```python
from build123d import *

# Parameters (mm, degrees)
BOSS_EXTRUDE1_DEPTH = 60
CUT_EXTRUDE2_DEPTH  = 25.152414984
BOSS_EXTRUDE2_DEPTH = 15
CUT_EXTRUDE3_DEPTH  = 25.152414984
BOSS_EXTRUDE3_DEPTH = 15
BOSS_EXTRUDE4_DEPTH = 15
CUT_EXTRUDE4_DEPTH  = 25.152414984
FILLET1_R           = 2


with BuildPart() as part:
    # Sketch1 → Boss-Extrude1 (new body)
    with BuildSketch(Plane.XY):
        Polygon((4.05, 18), (-124.05, 18), (-124.05, 0), (-115.95, 0), (-115.95, 3), (-4.05, 3), (-4.05, 0), (-7.95, 0), (-7.95, -2.04), (-4.048, -6.152414984), (4.048, -6.152414984), (7.95, -2.04), (7.95, 0), (4.05, 0), align=None)
    extrude(amount=BOSS_EXTRUDE1_DEPTH)

    # Sketch2 → Cut-Extrude2 (cut, through all)
    with BuildSketch(Plane(origin=(0, 18, 0), x_dir=(1, 0, 0), z_dir=(0, 1, 0))):
        Polygon((4.05, -60), (4.05, -6.625542325), (-109.904467136, -60), align=None)
        Polygon((-124.05, -60), (4.05, 0), (-124.05, 0), align=None)
        Polygon((11.122904285, -3.312706594), (4.05, -6.625542325), (4.05, -60), (-109.904467136, -60), (-126.032958173, -67.554328354), (-83.616740574, -158.112952928), (53.539121883, -93.871331168), align=None)
    extrude(amount=-CUT_EXTRUDE2_DEPTH, mode=Mode.SUBTRACT)

    # Sketch3 → Boss-Extrude2 (add, symmetric)
    with BuildSketch(Plane.XY.offset(60)):
        Polygon((-124.05, 18), (-124.05, 0), (-127.95, 0), (-127.95, -2.04), (-124.048, -6.152414984), (-115.952, -6.152414984), (-112.05, -2.04), (-112.05, 0), (-115.95, 0), (-115.95, 3), (-115.95, 18), align=None)
    extrude(amount=BOSS_EXTRUDE2_DEPTH, both=True)

    # Sketch2<4> → Cut-Extrude3 (cut, through all)
    with BuildSketch(Plane(origin=(0, 18, 0), x_dir=(1, 0, 0), z_dir=(0, 1, 0))):
        Polygon((4.05, 0), (-128.577931229, -62.12081088), (-170.994148827, 28.437813693), (-38.366217599, 90.558624573), align=None)
    extrude(amount=-CUT_EXTRUDE3_DEPTH, mode=Mode.SUBTRACT)

    # Sketch4 → Boss-Extrude3 (add)
    with BuildSketch(Plane(origin=(0, 18, 0), x_dir=(1, 0, 0), z_dir=(0, 1, 0))):
        Polygon((-109.904467136, -60), (-115.95, -62.831631318), (-115.95, -60), align=None)
    extrude(amount=-BOSS_EXTRUDE3_DEPTH)

    # Sketch6 → Boss-Extrude4 (add, symmetric)
    with BuildSketch(Plane(origin=(0, 0, 0), x_dir=(-1, 0, 0), z_dir=(0, 0, -1))):
        Polygon((-4.05, 0), (-7.95, 0), (-7.95, -2.04), (-4.05, -6.150307134), (4.048, -6.152414984), (7.95, -2.04), (7.95, 0), (4.05, 0), (4.05, 3), (4.05, 18), (-4.05, 18), align=None)
    extrude(amount=BOSS_EXTRUDE4_DEPTH, both=True)

    # Sketch7 → Cut-Extrude4 (cut, through all)
    with BuildSketch(Plane(origin=(0, 18, 0), x_dir=(1, 0, 0), z_dir=(0, 1, 0))):
        Polygon((-7.95, -12.246151224), (-7.95, -15), (7.95, -15), (7.95, -4.798844433), align=None)
    extrude(amount=-CUT_EXTRUDE4_DEPTH, mode=Mode.SUBTRACT)

    # Fillet1
    fillet1_edges = [part.edges().sort_by_distance(p)[0] for p in [
        (-115.95, 10.5, 62.831631318),
        (-4.05, 10.5, 3.793911007),
    ]]
    fillet(fillet1_edges, radius=FILLET1_R)


solid = part.part
```
For this review, take the finished solid that the model builds, in its own axes (mm). A direction names the side the tool comes from. Coordinates: 2 decimals unless noted, no trailing zeros. Order: outer loops, then holes, each group sorted by start corner. A loop starts at its lowest first (then second) coordinate and runs counter-clockwise, first axis right, second up. Notation, with made-up numbers: (-38.75, 43) -> (-0.75, 43) arc R19 ccw to (-0.75, 65) -> close; hole circle Ø9 at (-30.5, 39). An arc over 180 degrees is marked (long way). Answer as CSV lines item,"result".
Q1. Wall thickness on line 1 along X through (y, z) = (4.25, 70); line 2 along X through (y, z) = (16, -5); line 3 along Z through (x, y) = (-66.5, 14.25): over which ranges is each line inside the solid? List them lowest first. Write a range as [from, to].
Model answer:
line 1,"x = [-124.05, -115.95]"
line 2,"x = [-4.05, 4.05]"
line 3,"z = [33.04, 39.67]"
Q2. Clearance check with flat-ended pins moving along their axes: pin 1 Ø1.5 at (x, y) = (-104, 3.5) entering from +Z; pin 2 Ø10 at (y, z) = (2, 37.5) entering from -X; pin 3 Ø2 at (x, z) = (-113.5, 65.5) entering from +Y. State where each tip first meets the part, or that it passes through.
Model answer:
pin 1,"stops at z = 57.59"
pin 2,"stops at x = -86.47"
pin 3,"stops at y = 0"
Q3. For faces 1 (the face through (-126, 0, 68)), 2 (the face through (-114, 0, 65)), 3 (the face through (-56, 18, 30)), 4 (the face through (6, 0, -4)), 5 (the face through (-115.95, 7, 68)), list the 3-axis set-ups (+Z, -Z, +X, -X, +Y, -Y) from which the entire face can be reached by the end or side of a thin tool; tool diameter is ignored.
Model answer:
face 1,"+Z, -Z, -X, +Y"
face 2,"+Z, -Z, +X"
face 3,"+Z, -Z, +X, -X, +Y"
face 4,"+Z, -Z, +X, +Y"
face 5,"+Z, +X"
Q4. We need section B-B (x = -30). State the section outline as (y, z) points, plus the area to 3 significant figures.
Model answer:
outline,"(3, 15.95) -> (18, 15.95) -> (18, 22.57) -> (3, 22.57) -> close"
area,"99.4 mm2"
Q5. We need section C-C (z = 35). State the section outline as (x, y) points (3 decimals).
Model answer:
outline,"(-70.675, 3) -> (-56.529, 3) -> (-56.529, 18) -> (-70.675, 18) -> close"
Q6. We need section A-A (y = 14.5). State the section outline as (x, z) points.
Model answer:
outline,"(-124.05, 60) -> (-5.2, 4.33) arc R2 cw to (-4.05, 2.52) -> (-4.05, -15) -> (4.05, -15) -> (4.05, 6.63) -> (-114.8, 62.29) arc R2 cw to (-115.95, 64.1) -> (-115.95, 75) -> (-124.05, 75) -> close"
